Can you work these out from the drawing? Everything is in mm from the part's minimum corner. A direction names the side the tool comes from. Coordinates: 2 decimals unless noted, no trailing zeros. Order: outer loops, then holes, each group sorted by start corner. A loop starts at its lowest first (then second) coordinate and runs counter-clockwise, first axis right, second up. Notation, with made-up numbers: (-35.5, 64.25) -> (-12.5, 64.25) arc R30 cw to (-12.5, 101.25) -> close; hole circle Ø4 at (-0.5, 20.5). An arc over 180 degrees is marked (long way). Write item = value, one per line. Start each with the question number.
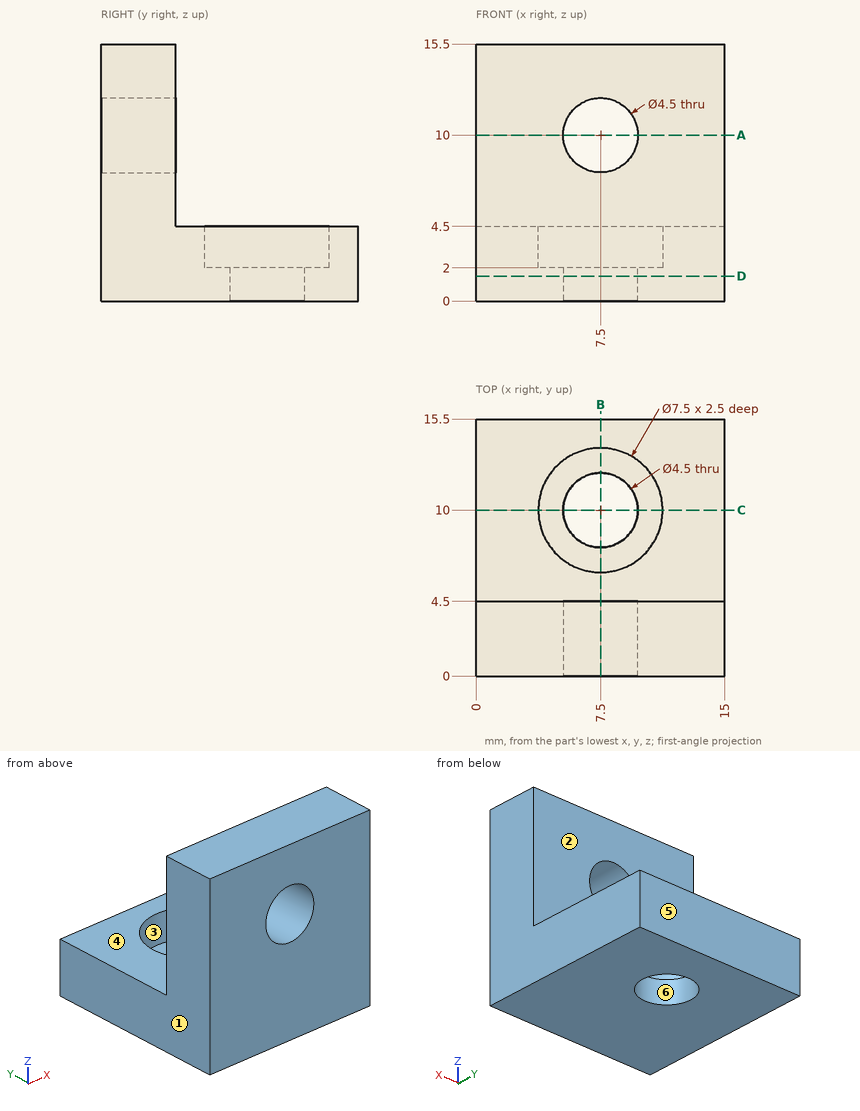
(1) For P1, Ø1.5, axis at x = 6.5, z = 11.5, coming from the +Y side; P2, Ø9, axis at x = 11, y = 10, coming from the +Z side; P3, Ø4, axis at y = 13.5, z = 8, coming from the -X side; P4, Ø4, axis at x = 8, y = 9, coming from the +Z side, each with a flat end and sliding along its axis, tell me the tip position at first contact or that it passes through.
(2) For the marked faces 1, 2 and 3, which set-ups out of +Z, -Z, +X, -X, +Y, -Y let a thin tool reach every point of the face, with its end or its side?
(3) If I drill on L1, parallel to X at y = 10, z = 1.55; L2, parallel to Y at x = 7.5, z = 1.4; L3, parallel to Z at x = 5, y = 13.5, over which ranges is the centre line in solid material (lowest first)? Write a range as from..to.
(4) Imagine slicing it at A-A (z = 10). Write out the boundary of the cut face in (x, y), plus the area to 4 significant figures.
(5) Imagine slicing it at D-D (z = 1.5). Write out the boundary of the cut face in (x, y).
(6) Thinking about a two-plate mould opening in Y: for the marked faces 4, 5 and 6, which applies, +Y half, -Y half, draft (parallel to the pull), parting line (faces both ways), or undercut?
(7) Imagine slicing it at B-B (x = 7.5). Write out the boundary of the cut face in (y, z).
(8) Imagine slicing it at C-C (y = 10). Write out the boundary of the cut face in (x, z), plus the area to 4 significant figures.
Result set:
q1.P1 = 4.5
q1.P2 = 4.5
q1.P3 = through
q1.P4 = 2
q2.face_1 = +Z, -Z, -X, +Y, -Y
q2.face_2 = +Z, +X, -X, +Y
q2.face_3 = +Z
q3.L1 = 0..5.25, 9.75..15
q3.L2 = 0..7.75, 12.25..15.5
q3.L3 = 0..4.5
q4.outline = (0, 0) -> (5.25, 0) -> (5.25, 4.5) -> (0, 4.5) -> close; (9.75, 0) -> (15, 0) -> (15, 4.5) -> (9.75, 4.5) -> close
q4.area = 47.25 mm2
q5.outline = (0, 0) -> (15, 0) -> (15, 15.5) -> (0, 15.5) -> close; hole circle Ø4.5 at (7.5, 10)
q6.face_4 = draft
q6.face_5 = +Y half
q6.face_6 = undercut
q7.outline = (0, 0) -> (7.75, 0) -> (7.75, 2) -> (6.25, 2) -> (6.25, 4.5) -> (4.5, 4.5) -> (4.5, 7.75) -> (0, 7.75) -> close; (0, 12.25) -> (4.5, 12.25) -> (4.5, 15.5) -> (0, 15.5) -> close; (12.25, 0) -> (15.5, 0) -> (15.5, 4.5) -> (13.75, 4.5) -> (13.75, 2) -> (12.25, 2) -> close
q8.outline = (0, 0) -> (5.25, 0) -> (5.25, 2) -> (3.75, 2) -> (3.75, 4.5) -> (0, 4.5) -> close; (9.75, 0) -> (15, 0) -> (15, 4.5) -> (11.25, 4.5) -> (11.25, 2) -> (9.75, 2) -> close
q8.area = 39.75 mm2
